For this review, use the dimensioned drawing (mm, ordinates from the lowest corner) and the shaded views. A direction names the side the tool comes from. Give positions to 0.01 mm unless a question says otherwise; leave off trailing zeros. Order: outer loops, then holes, each group sorted by start corner. A loop starts at its lowest first (then second) coordinate and runs counter-clockwise, first axis right, second up. Notation, with made-up numbers: M -11,82.25 L 42,82.25 A28 ccw 42,102.25 Z; hole C 46.5,76 d3. An arc over 180 degrees is marked long. Answer as CSV lines item,"result". Start each with the question number.
1. Clearance check with a flat-ended pin moving along its axis: P1, Ø4, axis at y = 7, z = 3, coming from the -X side. State where the tip first meets the part, or that it passes through.
2. Machinability: for the marked faces 1 and 2, which of the approach directions +Z, -Z, +X, -X, +Y, -Y give a long, thin tool a straight path to every point of the face, cutting with its end or side? Answer none if there is none.
3. We need section A-A, the plane y = 4.15. Give the boundary of the cut face in (x, z).
4. We need section C-C, the plane z = 2.75. Give the boundary of the cut face in (x, y).
5. For line 1 along Y through (x, z) = (4, 5); line 2 along Z through (x, y) = (2.5, 8), list the stretches that pass through material, from the lowest coordinate up.
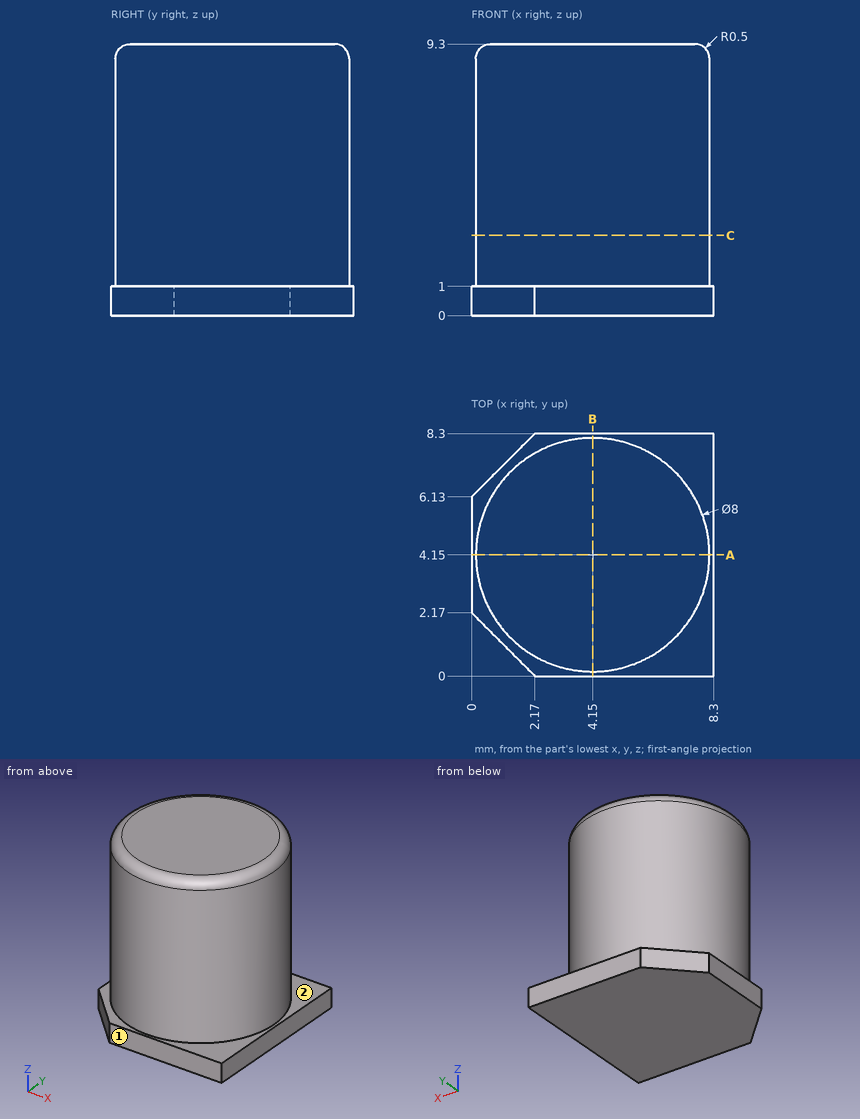
Result set:
1,P1,"x = 0.24"
2,face 1,"+Z, -Z, +X, -X, -Y"
2,face 2,"+Z"
3,outline,"M 0,0 L 8.3,0 L 8.3,1 L 8.15,1 L 8.15,8.8 A0.5 ccw 7.65,9.3 L 0.65,9.3 A0.5 ccw 0.15,8.8 L 0.15,1 L 0,1 Z"
4,outline,"C 4.15,4.15 d8"
5,line 1,"0.15 to 8.15"
5,line 2,"0 to 1"
